Could you check a few things on this model? Use its own coordinates, in mm. A direction names the side the tool comes from. Give positions to 0.01 mm unless a question says otherwise; leave off trailing zeros. Loops run counter-clockwise (first coordinate to the right, second up) from the corner with the lowest first, then second, coordinate; pieces in that order, holes last. Notation, with made-up numbers: (52, 45.25) - (78, 45.25) arc R23 ccw to (78, 67.25) - close; hole circle Ø4 at (-17.5, -5.75). An arc over 180 degrees is marked (long way). One line per item, written item: value. Start each with the question number.
Q1. If I drill on line 1 (Z direction, x = 0, y = 1.8); line 2 (Z direction, x = 0, y = 1.65); line 3 (Y direction, x = -3.5, z = -2), over which ranges is the centre line in solid material (lowest first)? Write a range as from..to.
Q2. I'm going to push flat-ended pins straight in: P1, Ø2, axis at x = 8, z = 0, coming from the +Y side; P2, Ø1.2, axis at x = 0, z = -7.5, coming from the -Y side (3 decimals); P3, Ø4, axis at x = -9, z = -9.5, coming from the -Y side. Where does each tip first touch, or does it pass through?
Q3. For faces 1 (the face through (0, 34, -2)), 2 (the face through (0, 43.18, 0)), 3 (the face through (-0.27, 1.57, 6.78)), which set-ups out of +Z, -Z, +X, -X, +Y, -Y let a thin tool reach every point of the face, with its end or its side?
Q4. If we mould it in two halves opening along X, with no side actions, what happens to faces 4 (the face through (-13.325, 13.241, 4.196)), 5 (the face through (-8, 3.175, 0)), 6 (the face through (0, 0, 0))? For each: released by +X, released by -X, zero draft, split by the parting line, or undercut.
Q5. I want a section at A-A (y = 28). Please give me the cut outline in (x, z).
Autodesk Inventor part; units mm, degrees
ref_plane "YZ Plane" through (0, 0, 0) normal (1, 0, 0) x (0, 1, 0)
ref_plane "XZ Plane" through (0, 0, 0) normal (0, 1, 0) x (-1, 0, 0)
ref_plane "XY Plane" through (0, 0, 0) normal (0, 0, 1) x (1, 0, 0)
sketch "Sketch1" plane through (0, 0, 0) normal (0, 0, 1) x (1, 0, 0)
  line L0 (0, 43.18) -> (0, 0)
  line L1 (-10.3763, 25.4) -> (-2, 25.4)
  line L2 (-2, 25.4) -> (-2, 43.18)
  line L3 (-2, 43.18) -> (0, 43.18)
  line L4 (0, 0) -> (-10.3763, 0)
  line L5 (-10.3763, 0) -> (-13.97, 3.466)
  line L6 (-13.97, 3.466) -> (-13.97, 22.9252)
  line L7 (-13.97, 22.9252) -> (-10.3763, 25.4)
  point P0 (0, 21.59)
  dimension "d18" = 2
  dimension "d19" = 17.78
  dimension "d23" = 25.4
  dimension "d25" = 13.97
revolve "Revolution1" add sketch "Sketch1" angle 360 about axis through (0, 43.18, 0) along (0, -1, 0)
fillet "Fillet3" radius 1.5875 1 edges at (10.3763, 25.4, 0)
fillet "Fillet4" radius 1.5875 1 edges at (13.97, 22.9252, 0)
fillet "Fillet5" radius 1.5875 2 edges at (13.97, 3.466, 0) (10.3763, 0, 0)
sketch "Sketch2" plane through (0, 0, 0) normal (0, -1, 0) x (1, 0, 0)
  circle A0 centre (0, 0) radius 9.7355
  circle A1 centre (8, 0) radius 1.25
  circle A2 centre (0, 8) radius 1.25
  circle A3 centre (-8, 0) radius 1.25
  circle A4 centre (0, -8) radius 1.25
  dimension "d29" = 2.5
  dimension "d32" = 360
  dimension "d36" = 8
extrude "Extrusion1" cut sketch "Sketch2" against normal blind 3.175 contours A1 | A2 | A3 | A4
properties part number "MotorTop"
Worked answers:
1. line 1: z = -12.24..-9.25, -6.75..6.75, 9.25..12.24
1. line 2: z = -12.09..-9.25, -6.75..6.75, 9.25..12.09
1. line 3: y = 0..25.4
2. P1: stops at y = 25.4
2. P2: stops at y = 3.175
2. P3: stops at y = 0.68
3. face 1: +Y
3. face 2: +Z, -Z, +X, -X, +Y
3. face 3: -Y
4. face 4: split by the parting line
4. face 5: undercut
4. face 6: zero draft
5. outline: circle Ø4 at (0, 0)
